For this review, take the finished solid that the model builds, in its own axes (mm). Face numbers are marked on the shaded views. Round coordinates to 2 decimals unless told otherwise and drop trailing zeros. Order: outer loops, then holes, each group sorted by start corner. A loop starts at its lowest first (then second) coordinate and runs counter-clockwise, first axis right, second up. Notation, with made-up numbers: M 89.25,87.25 L 127.25,87.25 A9 cw 127.25,97.25 Z; hole C -31,86.5 d6. An arc over 180 degrees is marked long. Answer in a Markdown table with one row per item. Add a question column.
```python
from build123d import *

# Parameters (mm, degrees)
BOSS_EXTRUDE1_DEPTH    = 3.175
F_10_CLEARANCE_HOLE1_D = 4.9784


with BuildPart() as part:
    # Sketch4 → Boss-Extrude1 (new body)
    with BuildSketch(Plane.XY):
        Polygon((-42.188928966, 293.919436917), (-7.296735047, 282.582275868), (-7.296735047, 248.458198081), (-18.653675695, 248.458198081), (-46.113444794, 283.07832781), align=None)
    extrude(amount=BOSS_EXTRUDE1_DEPTH)

    # #10 Clearance Hole1 (through all)
    with Locations(Plane.XY.offset(3.175)):
        with Locations((-32.740251946, 283.138719963), (-14.622625311, 277.25194622), (-14.622625311, 258.20194622)):
            Hole(F_10_CLEARANCE_HOLE1_D / 2)


solid = part.part
```
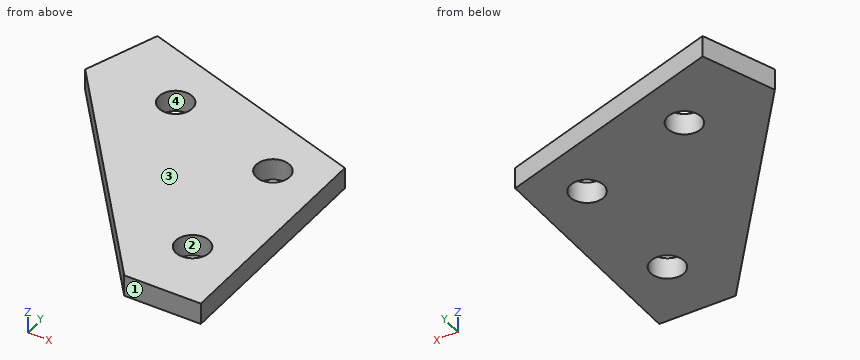
1. Consider section B-B on y = 276. Write out the cut boundary in (x, z) (3 decimals), plus the area to 3 significant figures.
2. The part is to be moulded in two halves that separate along Y. For the marked faces 1, 2, 3 and 4, say which applies: pulls with the +Y half, pulls with the -Y half, needs draft (parallel to the pull), parting line crosses it, or undercut.
3. Consider section C-C on z = 2.15. Write out the cut boundary in (x, y).
4. To check wall thickness, follow probe 1 along Y at (x, z) = (-15, 0.45); probe 2 along Y at (x, z) = (-33, 1); probe 3 along Y at (x, z) = (-11.5, 1.95). State the ranges of each line that lie inside material, in increasing order. Write a range as [from, to].
5. Consider section A-A on x = -34.5. Write out the cut boundary in (y, z) (3 decimals).
6. Consider section D-D on y = 252. Write out the cut boundary in (x, z) (3 decimals).
Solved:
| question | item | result |
|---|---|---|
| 1 | outline | M -40.499,0 L -16.774,0 L -16.774,3.175 L -40.499,3.175 Z; M -12.471,0 L -7.297,0 L -7.297,3.175 L -12.471,3.175 Z |
| 1 | area | 91.8 mm^2 |
| 2 | face 1 | pulls with the -Y half |
| 2 | face 2 | undercut |
| 2 | face 3 | needs draft |
| 2 | face 4 | undercut |
| 3 | outline | M -46.11,283.08 L -18.65,248.46 L -7.3,248.46 L -7.3,282.58 L -42.19,293.92 Z; hole C -32.74,283.14 d4.98; hole C -14.62,258.2 d4.98; hole C -14.62,277.25 d4.98 |
| 4 | probe 1 | y = [248.46, 255.74], [260.66, 274.79], [279.71, 285.09] |
| 4 | probe 2 | y = [266.55, 280.66], [285.61, 290.93] |
| 4 | probe 3 | y = [248.46, 283.95] |
| 5 | outline | M 268.437,0 L 281.378,0 L 281.378,3.175 L 268.437,3.175 Z; M 284.899,0 L 291.421,0 L 291.421,3.175 L 284.899,3.175 Z |
| 6 | outline | M -21.463,0 L -7.297,0 L -7.297,3.175 L -21.463,3.175 Z |
